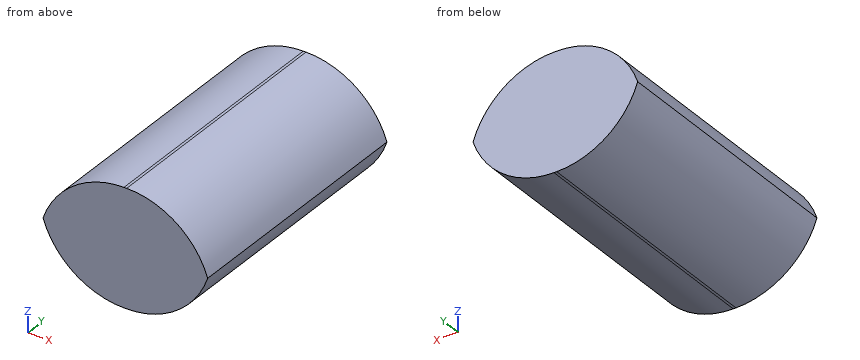
```python
from build123d import *

# Parameters (mm, degrees)
F0_W        = 27.7576074004
F0_H        = 41.3104146719
F1_DEPTH    = 18.6459105462
F2_T1_DEPTH = 109.6348425509


# Not quite as in the source:
# - a fillet or chamfer that OpenCascade refuses, or shapes differently, is made with other operations: its cross-section is extruded or revolved along the edge and cut away or added


with BuildPart() as f1:
    # F0 (on Top) → F1 (new body)
    with BuildSketch(Plane.XY):
        with Locations((27.7516692877, -49.2671057582)):
            Rectangle(F0_W, F0_H)
    extrude(amount=F1_DEPTH)

    # F2: fillet of radius 13.6648855758 on 4 edges, made by hand

    # F2_s2 → F2_t1 (cut)
    with BuildSketch(Plane.XZ.offset(-5.5503155173)):
        with BuildLine():
            ThreePointArc((41.6304729879, 4.9810249704), (37.6281206669, 14.6435582252), (27.9655874121, 18.6459105462))
            Line((27.9655874121, 18.6459105462), (41.6304729879, 18.6459105462))
            Line((41.6304729879, 18.6459105462), (41.6304729879, 4.9810249704))
        make_face()
        with BuildLine():
            ThreePointArc((13.8728655875, 4.9810249704), (17.8752179085, 14.6435582252), (27.5377511633, 18.6459105462))
            Line((27.5377511633, 18.6459105462), (13.8728655875, 18.6459105462))
            Line((13.8728655875, 18.6459105462), (13.8728655875, 4.9810249704))
        make_face()
        with BuildLine():
            ThreePointArc((41.6304729879, 13.6648855758), (37.6281206669, 4.002352321), (27.9655874121, 0))
            Line((27.9655874121, 0), (41.6304729879, 0))
            Line((41.6304729879, 0), (41.6304729879, 13.6648855758))
        make_face()
        with BuildLine():
            ThreePointArc((13.8728655875, 13.6648855758), (17.8752179085, 4.002352321), (27.5377511633, 0))
            Line((27.5377511633, 0), (13.8728655875, 0))
            Line((13.8728655875, 0), (13.8728655875, 13.6648855758))
        make_face()
    extrude(amount=F2_T1_DEPTH, mode=Mode.SUBTRACT)


solid = f1.part
```
Read the model definition and answer for the solid it produces. Units are mm, in the model's axes. Round coordinates to 2 decimals unless told otherwise and drop trailing zeros. Write each loop counter-clockwise with the first axis right and the second up, starting at its lowest first coordinate (ties: lowest second). Pieces come first, ordered by that corner, then holes. Notation, with made-up numbers: (34, 67) - (91, 67) arc R26 cw to (91, 94) - close; hole circle Ø1 at (52, 3). An arc over 180 degrees is marked (long way). One line per item, written item: value.
Q1. Find section C-C (z = 5.5). Determine the outline of the cut face in (x, y), and give its area (3 significant figures).
The answers:
outline: (16.58, -69.92) - (38.92, -69.92) - (38.92, -28.61) - (16.58, -28.61) - close
area: 923 mm2
Q2. Find section A-A (y = -41.5). Determine the outline of the cut face in (x, z), and give its area (3 significant figures).
The answers:
outline: (14.58, 9.32) arc R13.66 ccw to (27.54, 0) - (27.97, 0) arc R13.66 ccw to (40.92, 9.32) arc R13.66 ccw to (27.97, 18.65) - (27.54, 18.65) arc R13.66 ccw to start
area: 361 mm2
Q3. Straight lines are drawn through the part: line 1 (Z direction, x = 20, y = -64.5); line 2 (Z direction, x = 26.5, y = -52.5); line 3 (X direction, y = -56, z = 14). For each, find the intervals that lie inside material, in ascending order. Write a range as from..to.
The answers:
line 1: z = 2.27..16.38
line 2: z = 0.04..18.61
line 3: x = 17.27..38.23
Q4. Each of these flat-tipped pins is pushed along its axis until it touches: P1, Ø6, axis at y = -34, z = 12.5, coming from the +X side; P2, Ø3, axis at y = -63.5, z = 5.5, coming from the +X side; P3, Ø4, axis at x = 30.5, y = -39, coming from the +Z side. Where does it stop, or does it pass through?
The answers:
P1: stops at x = 40.86
P2: stops at x = 39.89
P3: stops at z = 18.64
Q5. Find section B-B (x = 34.5). Determine the outline of the cut face in (y, z), and give its area (3 significant figures).
The answers:
outline: (-69.92, 1.66) - (-28.61, 1.66) - (-28.61, 16.98) - (-69.92, 16.98) - close
area: 633 mm2
